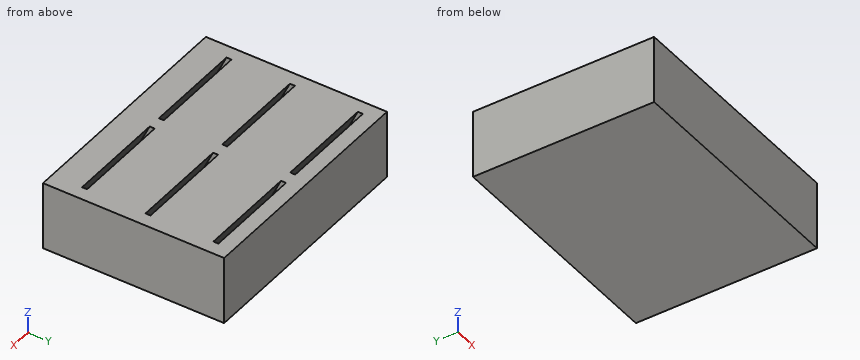
from build123d import *

# Parameters (mm, degrees)
BOX001_W               = 22
BOX001_H               = 1
BOX001_DEPTH           = 15
BOX001_PLACEMENT_ANGLE = 335
BOX003_W               = 22
BOX003_H               = 1
BOX003_DEPTH           = 15
BOX003_PLACEMENT_ANGLE = 335
BOX006_W               = 22
BOX006_H               = 1
BOX006_DEPTH           = 15
BOX006_PLACEMENT_ANGLE = 335
BOX002_W               = 22
BOX002_H               = 1
BOX002_DEPTH           = 15
BOX002_PLACEMENT_ANGLE = 335
BOX004_W               = 22
BOX004_H               = 1
BOX004_DEPTH           = 15
BOX004_PLACEMENT_ANGLE = 335
BOX005_W               = 22
BOX005_H               = 1
BOX005_DEPTH           = 15
BOX005_PLACEMENT_ANGLE = 335
BOX_W                  = 53
BOX_H                  = 40
BOX_DEPTH              = 15


with BuildPart() as cube001:
    # Box001 → Box001 (new body)
    with BuildSketch(Plane.XY):
        with Locations((11, 0.5)):
            Rectangle(BOX001_W, BOX001_H)
    extrude(amount=BOX001_DEPTH)


with BuildPart() as cube001_1:
    # Box001 placement: moved
    add(cube001.part.moved(Location((3, 15, 3))).rotate(Axis((3, 15, 3), (1, 0, 0)), BOX001_PLACEMENT_ANGLE))


with BuildPart() as cube003:
    # Box003 → Box003 (new body)
    with BuildSketch(Plane.XY):
        with Locations((11, 0.5)):
            Rectangle(BOX003_W, BOX003_H)
    extrude(amount=BOX003_DEPTH)


with BuildPart() as cube003_1:
    # Box003 placement: moved
    add(cube003.part.moved(Location((3, 30, 3))).rotate(Axis((3, 30, 3), (1, 0, 0)), BOX003_PLACEMENT_ANGLE))


with BuildPart() as cube006:
    # Box006 → Box006 (new body)
    with BuildSketch(Plane.XY):
        with Locations((11, 0.5)):
            Rectangle(BOX006_W, BOX006_H)
    extrude(amount=BOX006_DEPTH)


with BuildPart() as cube006_1:
    # Box006 placement: moved
    add(cube006.part.moved(Location((28, 1, 3))).rotate(Axis((28, 1, 3), (1, 0, 0)), BOX006_PLACEMENT_ANGLE))


with BuildPart() as cube002:
    # Box002 → Box002 (new body)
    with BuildSketch(Plane.XY):
        with Locations((11, 0.5)):
            Rectangle(BOX002_W, BOX002_H)
    extrude(amount=BOX002_DEPTH)


with BuildPart() as cube002_1:
    # Box002 placement: moved
    add(cube002.part.moved(Location((28, 15, 3))).rotate(Axis((28, 15, 3), (1, 0, 0)), BOX002_PLACEMENT_ANGLE))


with BuildPart() as cube004:
    # Box004 → Box004 (new body)
    with BuildSketch(Plane.XY):
        with Locations((11, 0.5)):
            Rectangle(BOX004_W, BOX004_H)
    extrude(amount=BOX004_DEPTH)


with BuildPart() as cube004_1:
    # Box004 placement: moved
    add(cube004.part.moved(Location((28, 30, 3))).rotate(Axis((28, 30, 3), (1, 0, 0)), BOX004_PLACEMENT_ANGLE))


with BuildPart() as fusion:
    # Box005 → Box005 (new body)
    with BuildSketch(Plane.XY):
        with Locations((11, 0.5)):
            Rectangle(BOX005_W, BOX005_H)
    extrude(amount=BOX005_DEPTH)


with BuildPart() as fusion_1:
    # Box005 placement: moved
    add(fusion.part.moved(Location((3, 1, 3))).rotate(Axis((3, 1, 3), (1, 0, 0)), BOX005_PLACEMENT_ANGLE))

    # Fusion: union Cube001, Cube003, Cube006, Cube002, Cube004
    add(cube001_1.part)
    add(cube003_1.part)
    add(cube006_1.part)
    add(cube002_1.part)
    add(cube004_1.part)


with BuildPart() as cut:
    # Box → Box (new body)
    with BuildSketch(Plane.XY):
        with Locations((26.5, 20)):
            Rectangle(BOX_W, BOX_H)
    extrude(amount=BOX_DEPTH)

    # Cut: cut Fusion
    add(fusion_1.part, mode=Mode.SUBTRACT)


solid = cut.part
Here's how the part is built. I have some questions about the finished solid (model axes, mm). Coordinates: 2 decimals unless noted, no trailing zeros. Order: outer loops, then holes, each group sorted by start corner. A loop starts at its lowest first (then second) coordinate and runs counter-clockwise, first axis right, second up. Notation, with made-up numbers: M 65.5,72 L 99.5,72 A22 cw 99.5,111 Z; hole C -14.5,39.5 d5. An arc over 180 degrees is marked long. Answer as CSV lines item,"result". Start each with the question number.
1. For pin 1 (3.5 mm diameter, centred on y = 18.5, z = 11, fed in from -X), with a flat end and sliding along its axis, tell me the tip position at first contact or that it passes through.
2. I need wall thicknesses on line 1 (Y direction, x = 45, z = 3.25); line 2 (Y direction, x = 6.5, z = 13.5); line 3 (Z direction, x = 17, y = 2.5). Which ranges of each line are inside material? Lowest first, please. Write a range as [from, to].
3. I want a section at A-A, the plane y = 33. Write out the boundary of the cut face in (x, z), and give its area (3 significant figures).
4. I want a section at C-C, the plane z = 10.75. Write out the boundary of the cut face in (x, y), and give its area (3 significant figures).
5. I want a section at B-B, the plane x = 7.5. Write out the boundary of the cut face in (y, z).
Recorded:
1,pin 1,"stops at x = 0"
2,line 1,"y = [0, 1.12], [2.22, 15.12], [16.22, 30.12], [31.22, 40]"
2,line 2,"y = [0, 5.9], [7, 19.9], [21, 34.9], [36, 40]"
2,line 3,"z = [0, 3.85], [6.22, 15]"
3,outline,"M 0,0 L 53,0 L 53,15 L 0,15 Z; hole M 3,7.07 L 25,7.07 L 25,9.43 L 3,9.43 Z; hole M 28,7.07 L 50,7.07 L 50,9.43 L 28,9.43 Z"
3,area,"691 mm2"
4,outline,"M 0,0 L 53,0 L 53,40 L 0,40 Z; hole M 3,4.61 L 25,4.61 L 25,5.72 L 3,5.72 Z; hole M 3,18.61 L 25,18.61 L 25,19.72 L 3,19.72 Z; hole M 3,33.61 L 25,33.61 L 25,34.72 L 3,34.72 Z; hole M 28,4.61 L 50,4.61 L 50,5.72 L 28,5.72 Z; hole M 28,18.61 L 50,18.61 L 50,19.72 L 28,19.72 Z; hole M 28,33.61 L 50,33.61 L 50,34.72 L 28,34.72 Z"
4,area,"1,970 mm2"
5,outline,"M 0,0 L 40,0 L 40,15 L 36.7,15 L 30.91,2.58 L 30,3 L 35.6,15 L 21.7,15 L 15.91,2.58 L 15,3 L 20.6,15 L 7.7,15 L 1.91,2.58 L 1,3 L 6.6,15 L 0,15 Z"
